For this review, use the dimensioned drawing (mm, ordinates from the lowest corner) and the shaded views. Round coordinates to 2 decimals unless told otherwise and drop trailing zeros. Write each loop counter-clockwise with the first axis right and the second up, starting at its lowest first coordinate (ties: lowest second). Pieces come first, ordered by that corner, then holes. Notation, with made-up numbers: M 44.25,23 L 58.25,23 A20 cw 58.25,49 Z; hole C -24,70.5 d2. An arc over 180 degrees is marked long. One line per question, with ' | ' between items. Start each with the question number.
Item 1: Add section B-B, the plane z = 1123.5. State the section outline as (x, y) points.
Item 2: Add section C-C, the plane x = 459. State the section outline as (y, z) points.
Item 3: For L1, parallel to Y at x = 707.5, z = 214.5, list the stretches that pass through material, from the lowest coordinate up.
Item 4: Insertion check: pin 1 Ø5 at (x, z) = (1572.5, 927) entering from -Y. The pin has a flat end and moves straight along its axis. Give the tip position at first contact, or say it passes through.
Item 5: Add section A-A, the plane y = 765.5. Give the number of separate pieces and of enclosed holes in the cut face, and give its area (3 significant figures).
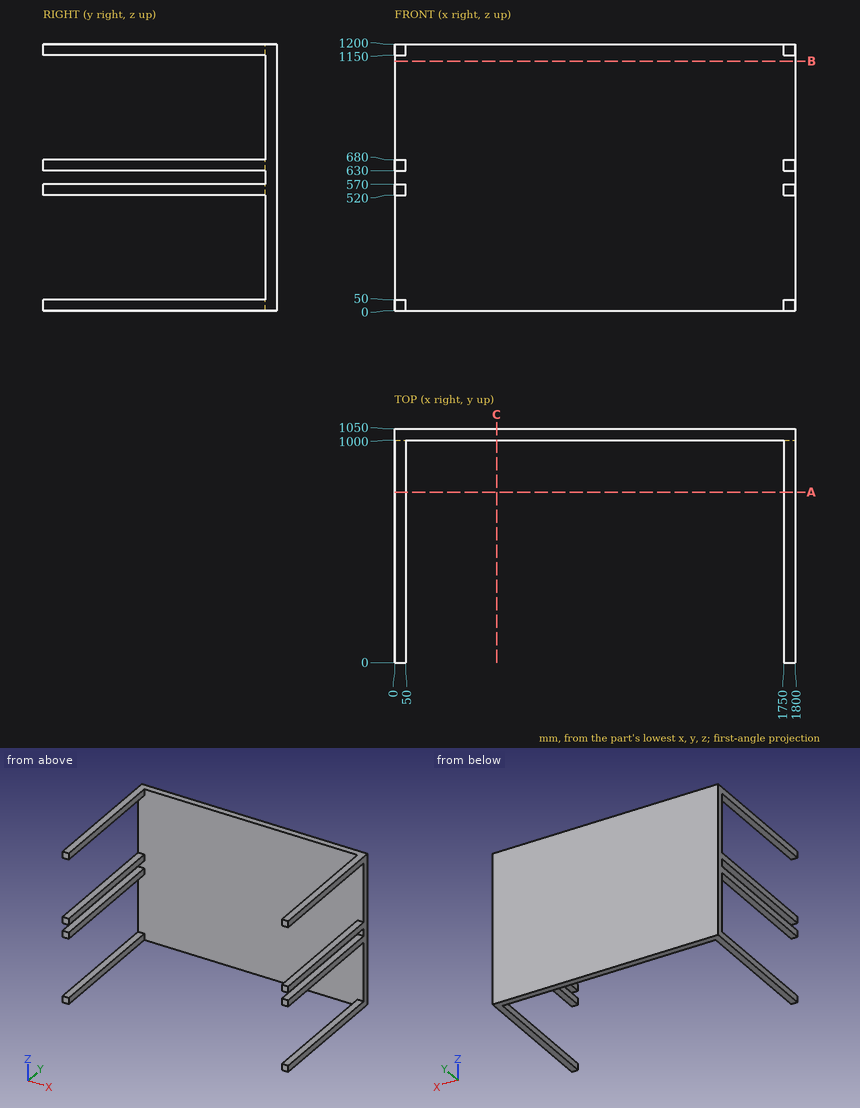
Computed values:
1) outline: M 0,1000 L 1800,1000 L 1800,1050 L 0,1050 Z
2) outline: M 1000,0 L 1050,0 L 1050,1200 L 1000,1200 Z
3) L1: y = 1000 to 1050
4) pin 1: stops at y = 1000
5) separate pieces: 8 | enclosed holes: 0 | area: 20,000 mm^2
